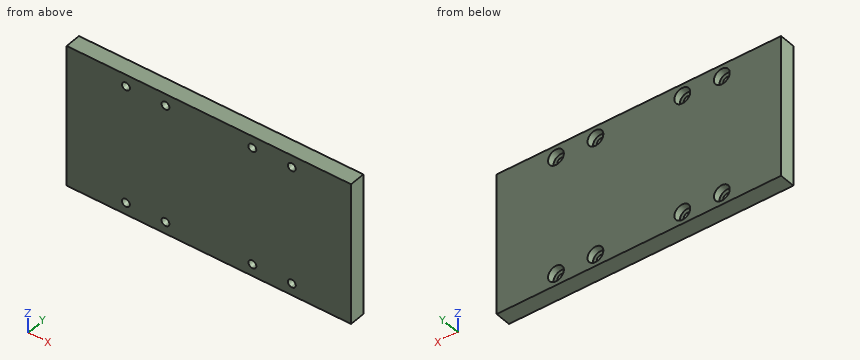
from build123d import *

# Parameters (mm, degrees)
SKETCH1_W           = 228.6
SKETCH1_H           = 114.3
BOSS_EXTRUDE1_DEPTH = 12.7
SKETCH2_R           = 3.175
CUT_EXTRUDE1_DEPTH  = 311.912
SKETCH3_R           = 6.35
CUT_EXTRUDE2_DEPTH  = 5.55625


with BuildPart() as part:
    # Sketch1 → Boss-Extrude1 (new body)
    with BuildSketch(Plane(origin=(0, 0, 0), x_dir=(1, 0, 0), z_dir=(0, 1, 0))):
        with Locations((114.3, 57.15)):
            Rectangle(SKETCH1_W, SKETCH1_H)
    extrude(amount=BOSS_EXTRUDE1_DEPTH)

    # Sketch2 → Cut-Extrude1 (cut)
    with BuildSketch(Plane.XZ):
        with Locations((47.625, -9.525)):
            Circle(SKETCH2_R)
        with Locations((79.375, -9.525)):
            Circle(SKETCH2_R)
        with Locations((149.225, -9.525)):
            Circle(SKETCH2_R)
        with Locations((180.975, -9.525)):
            Circle(SKETCH2_R)
        with Locations((47.625, -104.775)):
            Circle(SKETCH2_R)
        with Locations((79.375, -104.775)):
            Circle(SKETCH2_R)
        with Locations((149.225, -104.775)):
            Circle(SKETCH2_R)
        with Locations((180.975, -104.775)):
            Circle(SKETCH2_R)
    extrude(amount=-CUT_EXTRUDE1_DEPTH, mode=Mode.SUBTRACT)

    # Sketch3 → Cut-Extrude2 (cut)
    with BuildSketch(Plane(origin=(0, 12.7, 0), x_dir=(1, 0, 0), z_dir=(0, 1, 0))):
        with Locations((47.625, 104.775)):
            Circle(SKETCH3_R)
        with Locations((79.375, 104.775)):
            Circle(SKETCH3_R)
        with Locations((149.225, 104.775)):
            Circle(SKETCH3_R)
        with Locations((180.975, 104.775)):
            Circle(SKETCH3_R)
        with Locations((47.625, 9.525)):
            Circle(SKETCH3_R)
        with Locations((79.375, 9.525)):
            Circle(SKETCH3_R)
        with Locations((149.225, 9.525)):
            Circle(SKETCH3_R)
        with Locations((180.975, 9.525)):
            Circle(SKETCH3_R)
    extrude(amount=-CUT_EXTRUDE2_DEPTH, mode=Mode.SUBTRACT)


solid = part.part
Design review of the part built by this model. Coordinates are the model's own, in mm. Round coordinates to 2 decimals unless told otherwise and drop trailing zeros. Loops run counter-clockwise (first coordinate to the right, second up) from the corner with the lowest first, then second, coordinate; pieces in that order, holes last. Notation, with made-up numbers: M 2.5,-24.75 L 48.5,-24.75 A23 cw 48.5,-3.75 Z; hole C -19,66 d7. An arc over 180 degrees is marked long. Answer as a JSON object with one key per item and string values.
Item 1: We need section A-A on x = 48.5. Give the boundary of the cut face in (y, z), and give its area (3 significant figures).
Answer sheet:
{"outline": "M 0,-114.3 L 12.7,-114.3 L 12.7,-111.06 L 7.14,-111.06 L 7.14,-107.83 L 0,-107.83 Z; M 0,-101.72 L 7.14,-101.72 L 7.14,-98.49 L 12.7,-98.49 L 12.7,-15.81 L 7.14,-15.81 L 7.14,-12.58 L 0,-12.58 Z; M 0,-6.47 L 7.14,-6.47 L 7.14,-3.24 L 12.7,-3.24 L 12.7,0 L 0,0 Z", "area": "1,220 mm^2"}
Item 2: Wall thickness on L1, parallel to Z at x = 84, y = 10; L2, parallel to Y at x = 148, z = -4.5: over which ranges is each line inside the solid? List them lowest first. Write a range as from..to.
Answer sheet:
{"L1": "z = -114.3..-109.13, -100.42..-13.88, -5.17..0", "L2": "y = 0..7.14"}
Item 3: Clearance check with a flat-ended pin moving along its axis: P1, Ø6.5, axis at x = 183, z = -10, coming from the +Y side. State where the tip first meets the part, or that it passes through.
Answer sheet:
{"P1": "stops at y = 7.14"}
Item 4: We need section B-B on y = 9.25. State how many separate pieces and enclosed holes the cut face has, and give its area (3 significant figures).
Answer sheet:
{"separate pieces": "1", "enclosed holes": "8", "area": "25,100 mm^2"}
